The model under review builds one solid part; all positions refer to its coordinate system, in mm. Coordinates: 2 decimals unless noted, no trailing zeros. Write each loop counter-clockwise with the first axis right and the second up, starting at its lowest first coordinate (ties: lowest second). Pieces come first, ordered by that corner, then holes. Notation, with made-up numbers: (61, 88.5) - (100, 88.5) arc R30 ccw to (100, 120.5) - close; hole circle Ø6 at (-2, -17.5). An arc over 180 degrees is marked (long way). Answer as CSV lines item,"result". Start each with the question number.
Autodesk Inventor part; units mm, degrees
ref_plane "Work Plane1" through (29, 0, 0) normal (0, -1, 0) x (1, 0, 0)
ref_plane "YZ Plane" through (0, 0, 0) normal (1, 0, 0) x (0, 1, 0)
ref_plane "XZ Plane" through (0, 0, 0) normal (0, 1, 0) x (-1, 0, 0)
sketch "Sketch1" plane through (0, 0, 0) normal (0, 0, 1) x (1, 0, 0)
  line L0 (0, 0) -> (6, 0)
  line L1 (6, 0) -> (6, 1)
  line L2 (6, 1) -> (1.5, 1)
  line L3 (1.5, 1) -> (1.1932, 1)
  line L4 (1.1932, 1) -> (0, 1)
  line L5 (0, 1) -> (0, 1.75)
  line L6 (0, 1.75) -> (-1.2, 1.75)
  line L7 (-1.2, 1.75) -> (-1.2, 0.866)
  line L8 (-1.2, 0.866) -> (-0.5, 0.866)
  line L9 (-0.5, 0.866) -> (0, 0)
  line L10 (-2.64, 0) -> (7.44, 0)
  line L11 (0, -0.35) -> (0, 2.1)
  line L12 (1.5, 1) -> (0, 1) construction
  dimension "d1" = 4.5
  dimension "d2" = 0.3068
  dimension "d3" = 1.2
  dimension "d4" = 0.7
  dimension "d5" = 60
  dimension "d6" = 2
  dimension "d7" = 2
  dimension "d8" = 1.7321
  dimension "d9" = 3.5
  dimension "d26" = 6
revolve "Body" add sketch "Sketch1" angle 360 about axis through (0, 0, 0) along (1, 0, 0)
sketch "Sketch2" plane through (-1.2, 0, 0) normal (-1, 0, 0) x (0, 0, 1)
  circle A0 centre (0, 0) radius 0.866
  line L0 (0, -2.45) -> (0, 2.45)
  line L1 (-2.45, 0) -> (2.45, 0)
  line L2 (0.866, 0) -> (0.433, -0.75)
  line L3 (0.433, -0.75) -> (-0.433, -0.75)
  line L4 (-0.433, -0.75) -> (-0.866, 0)
  line L5 (-0.866, 0) -> (-0.433, 0.75)
  line L6 (-0.433, 0.75) -> (0.433, 0.75)
  line L7 (0.433, 0.75) -> (0.866, 0)
extrude "Slot" add sketch "Sketch2" against normal up to next contours L7 A0 | A0 L2 | L6 L0 A0 | A0 L0 L3 | L0 L6 A0 | A0 L3 L0 | L4 A0 | A0 L5
fillet "Fillet1" radius 0.8 1 edges at (-1.2, -1.75, 0)
chamfer "Chamfer1" distance 0.3067 distance2 0.3067 1 edges at (6, -1, 0) measured on face at (6, 0.1182, 0.3117)
ref_plane "Work Plane1" through (29, 0, 0) normal (0, -1, 0) x (1, 0, 0)
fillet "Fillet2" radius 0.1 1 edges at (0, -1, 0)
thread "Thread2"
equation "\"d15\" = -0.5 * SPD + 0.5 * GD"
equation "\"d16\" = GUL"
equation "\"d1\" = GEL"
equation "\"GD\" = NND"
equation "\"NLG\" = 6"
equation "\"GEL\" = 4.5"
equation "\"KOD\" = 5.7"
equation "\"KOH\" = 1.65"
equation "\"INTI\" = 1.04"
equation "\"GAL\" = 0.61345 * PTC"
equation "\"GUL\" = 0.61345 * PTC"
equation "\"BDM\" = NND"
equation "\"SW\" = 2"
equation "\"RR\" = 1.45"
equation "\"SPD\" = NND - 1.2269 * PTC"
equation "\"R\" = 0.3"
equation "\"TOA\" = 30deg"
equation "\"GD1\" = THREADDIA - 1.2269 * PTC"
equation "\"THREADDIA\" = 3"
equation "\"PTC\" = 0.5"
equation "\"NND\" = 3"
equation "\"KOH1\" = 0.2"
equation "\"E0\" = 2.303"
properties part number "ISO 7380-1 - M3 x 6" material "Stainless Steel"
(1) For pin 1 (2 mm diameter, centred on x = 3, y = 0, fed in from -Z); pin 2 (0.8 mm diameter, centred on x = -1, z = 0, fed in from +Y); pin 3 (1.5 mm diameter, centred on x = 2, z = 1.5, fed in from -Y), all flat-tipped, find the tip position at first contact; note any pin that passes through.
(2) Wall thickness on line 1 (Z direction, x = -0.5, y = 0.6); line 2 (Y direction, x = -0.5, z = 0.05); line 3 (Z direction, x = 4.25, y = 0.7): over which ranges is each line inside the solid? List them lowest first.
(3) Add section A-A on x = 1.5. Give the boundary of the cut face in (y, z), then the cut area to 3 significant figures.
(4) The part is to be moulded in two halves that separate along Z. For faces 1 (the cylindrical face through (-0.203, 1.617, 0.67)), 2 (the flat face through (6, 0, 0)), 3 (the conical face through (0, 0, 0)), say which applies: released by +Z, released by -Z, zero draft, split by the parting line, or undercut.
Reported:
1,pin 1,"z = -1"
1,pin 2,"y = 1.72"
1,pin 3,"y = -0.66"
2,line 1,"-1.64 to -0.52, 0.52 to 1.64"
2,line 2,"-1.74 to -0.75, 0.75 to 1.74"
2,line 3,"-0.71 to 0.71"
3,outline,"circle Ø2 at (0, 0)"
3,area,"3.14 mm²"
4,face 1,"split by the parting line"
4,face 2,"zero draft"
4,face 3,"undercut"
